Could you check a few things on this model? Use its own coordinates, in mm. A direction names the side the tool comes from. Give positions to 0.01 mm unless a question says otherwise; leave off trailing zeros. Loops run counter-clockwise (first coordinate to the right, second up) from the corner with the lowest first, then second, coordinate; pieces in that order, holes last. Notation, with made-up numbers: (60.25, 35) - (79.25, 35) arc R23 ccw to (79.25, 47) - close; hole circle Ø1 at (-16, -23). An arc over 180 degrees is marked (long way). One line per item, written item: value. Start each with the question number.
Q1. I want a section at C-C (z = 1.85). Please give me the cut outline in (x, y).
Q2. If we mould it in two halves opening along Y, with no side actions, what happens to faces 4 (the face through (10, -12, 2)), 5 (the face through (-55, 0, 1)), 6 (the face through (0, -20, 1)), 7 (the face through (-10, -12, 2))? For each: released by +Y, released by -Y, zero draft, split by the parting line, or undercut.
Q3. I'm going to push flat-ended pins straight in: P1, Ø4.5, axis at x = -10, y = 10, coming from the -Z side; P2, Ø3.5, axis at x = 10, y = 10, coming from the -Z side; P3, Ø1, axis at y = -15, z = 1.5, coming from the -X side; P4, Ø1.5, axis at x = -28, z = 2.5, coming from the +Y side. Where does each tip first touch, or does it pass through?
Q4. For faces 1 (the face through (-13.5, -12, 1)), 2 (the face through (-27.908, -0.601, 1.521)), 3 (the face through (-13.5, 13, 1)), which set-ups out of +Z, -Z, +X, -X, +Y, -Y let a thin tool reach every point of the face, with its end or its side?
Q5. I want a section at D-D (x = -26). Please give me the cut outline in (y, z).
Q6. I want a section at B-B (x = -10). Please give me the cut outline in (y, z).
Q7. If I drill on line 1 (Y direction, x = 10, z = 2); line 2 (X direction, y = 10, z = 1.4); line 3 (X direction, y = -10.5, z = 2.4), over which ranges is the centre line in solid material (lowest first)? Write a range as from..to.
Q8. I want a section at A-A (y = 0). Please give me the cut outline in (x, z).
```python
from build123d import *

# Parameters (mm, degrees)
F1_DEPTH = 3
F2_D     = 4


with BuildPart() as f1:
    # F0 (on Top) → F1 (new body)
    with BuildSketch(Plane.XY):
        Polygon((-13.5, -20), (13.5, -20), (13.5, 20), (-13.5, 20), (-13.5, 5.2414399013), (-55, 5.2414399013), (-55, -4.7585600987), (-13.5, -4.7585600987), align=None)
    extrude(amount=F1_DEPTH)

    # F2 (through all)
    with Locations(Plane(origin=(0, 0, 0), x_dir=(1, 0, 0), z_dir=(0, 0, -1))):
        with Locations((-51, 0), (-26, 0), (-10, 10), (10, -10), (10, 10), (-10, -10)):
            Hole(F2_D / 2)


solid = f1.part
```
Worked answers:
1. outline: (-55, -4.76) - (-13.5, -4.76) - (-13.5, -20) - (13.5, -20) - (13.5, 20) - (-13.5, 20) - (-13.5, 5.24) - (-55, 5.24) - close; hole circle Ø4 at (-51, 0); hole circle Ø4 at (-26, 0); hole circle Ø4 at (-10, -10); hole circle Ø4 at (-10, 10); hole circle Ø4 at (10, -10); hole circle Ø4 at (10, 10)
2. face 4: undercut
2. face 5: zero draft
2. face 6: released by -Y
2. face 7: undercut
3. P1: stops at z = 0
3. P2: passes through
3. P3: stops at x = -13.5
3. P4: stops at y = 5.24
4. face 1: +Z, -Z, -X, -Y
4. face 2: +Z, -Z
4. face 3: +Z, -Z, -X, +Y
5. outline: (-4.76, 0) - (-2, 0) - (-2, 3) - (-4.76, 3) - close; (2, 0) - (5.24, 0) - (5.24, 3) - (2, 3) - close
6. outline: (-20, 0) - (-12, 0) - (-12, 3) - (-20, 3) - close; (-8, 0) - (8, 0) - (8, 3) - (-8, 3) - close; (12, 0) - (20, 0) - (20, 3) - (12, 3) - close
7. line 1: y = -20..-12, -8..8, 12..20
7. line 2: x = -13.5..-12, -8..8, 12..13.5
7. line 3: x = -13.5..-11.94, -8.06..8.06, 11.94..13.5
8. outline: (-55, 0) - (-53, 0) - (-53, 3) - (-55, 3) - close; (-49, 0) - (-28, 0) - (-28, 3) - (-49, 3) - close; (-24, 0) - (13.5, 0) - (13.5, 3) - (-24, 3) - close
